The drawing under review shows one solid part. Ordinate dimensions are in mm from its lowest x, y, z. Give positions to 0.01 mm unless a question says otherwise; leave off trailing zeros. Order: outer loops, then holes, each group sorted by start corner. A loop starts at its lowest first (then second) coordinate and runs counter-clockwise, first axis right, second up. Notation, with made-up numbers: (58.5, 49.5) -> (83.5, 49.5) arc R23 cw to (83.5, 65.5) -> close; hole circle Ø5 at (-18.5, -9.5). An arc over 180 degrees is marked (long way). One line per item, written item: value. Start each with the question number.
1) For pin 1 (12 mm diameter, centred on y = 68.5, z = 19, fed in from -X) (1 decimal); pin 2 (5 mm diameter, centred on x = 81, y = 81, fed in from -Z); pin 3 (3 mm diameter, centred on y = 52.5, z = 22.5, fed in from -X) (1 decimal), all flat-tipped, find the tip position at first contact; note any pin that passes through.
2) Wall thickness on line 1 along Z through (x, y) = (58, 21); line 2 along Y through (x, z) = (52, 15) (1 decimal); line 3 along Y through (x, z) = (45, 11) (1 decimal): over which ranges is each line inside the solid? List them lowest first. Write a range as from..to.
3) The part is to be moulded in two halves that separate along Y. For the marked faces 1, 2 and 3, say which applies: released by +Y, released by -Y, zero draft, split by the parting line, or undercut.
4) Consider section A-A (z = 31). State the section outline as (x, y) points (1 decimal), plus the area to 3 significant figures.
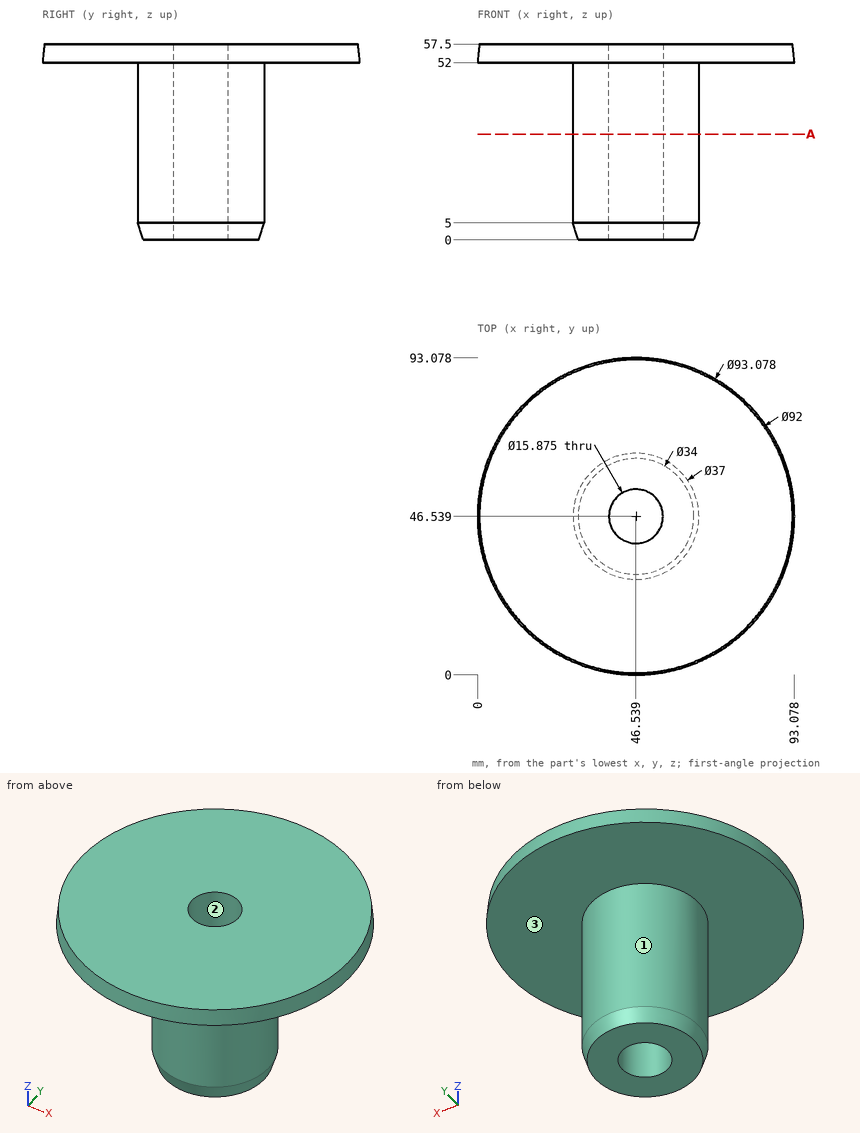
Checked values:
1. pin 1: stops at x = 37.2
1. pin 2: stops at z = 52
1. pin 3: stops at x = 28.6
2. line 1: z = 52..57.5
2. line 2: y = 28.9..40.8, 52.3..64.2
2. line 3: y = 28.1..38.8, 54.3..65
3. face 1: split by the parting line
3. face 2: undercut
3. face 3: zero draft
4. outline: circle Ø37 at (46.5, 46.5); hole circle Ø15.9 at (46.5, 46.5)
4. area: 877 mm^2
